from build123d import *

# Parameters (mm, degrees)
F0_W      = 340
F0_H      = 250
F1_DEPTH  = 220
F3_DEPTH  = 340
F4_R      = 110.000034
F5_DEPTH  = 228.6
F6_R      = 6.999986
F7_DEPTH  = 304.8
F8_W      = 75.12304
F8_H      = 29.99994
F9_DEPTH  = 2
F10_W     = 75
F10_H     = 30
F11_DEPTH = 2


with BuildPart() as f1:
    # F0 (on Front) → F1 (new body)
    with BuildSketch(Plane.XZ):
        Rectangle(F0_W, F0_H)
    extrude(amount=F1_DEPTH)

    # F2 (on face) → F3 (cut)
    with BuildSketch(Plane.YZ.offset(170)):
        with BuildLine():
            ThreePointArc((-40.00008, 89.98988), (-45.860908, 104.139172), (-60.0102, 110))
            Line((-60.0102, 110), (-159.98996, 110))
            ThreePointArc((-159.98996, 110), (-174.139252, 104.139172), (-180.00008, 89.98988))
            Line((-180.00008, 89.98988), (-180.00008, -89.98988))
            ThreePointArc((-180.00008, -89.98988), (-174.139252, -104.139172), (-159.98996, -110))
            Line((-159.98996, -110), (-60.0102, -110))
            ThreePointArc((-60.0102, -110), (-45.860908, -104.139172), (-40.00008, -89.98988))
            Line((-40.00008, -89.98988), (-40.00008, 89.98988))
        make_face()
    extrude(amount=-F3_DEPTH, mode=Mode.SUBTRACT)

    # F4 (on face) → F5 (cut)
    with BuildSketch(Plane.XZ.offset(220)):
        Circle(F4_R)
    extrude(amount=-F5_DEPTH, mode=Mode.SUBTRACT)

    # F6 (on face) → F7 (cut)
    with BuildSketch(Plane.XY.offset(125)):
        with Locations((0, -110.000034)):
            Circle(F6_R)
    extrude(amount=-F7_DEPTH, mode=Mode.SUBTRACT)

    # F8 (on face) → F9 (join)
    with BuildSketch(Plane(origin=(0, 0, -125), x_dir=(1, 0, 0), z_dir=(0, 0, -1))):
        with Locations((-132.43848, 205.00003)):
            Rectangle(F8_W, F8_H)
        with Locations((-132.43848, 14.99997)):
            Rectangle(F8_W, F8_H)
    extrude(amount=F9_DEPTH)

    # F10 (on face) → F11 (join)
    with BuildSketch(Plane(origin=(0, 0, -125), x_dir=(1, 0, 0), z_dir=(0, 0, -1))):
        with Locations((132.5, 110)):
            Rectangle(F10_W, F10_H)
    extrude(amount=F11_DEPTH)


solid = f1.part
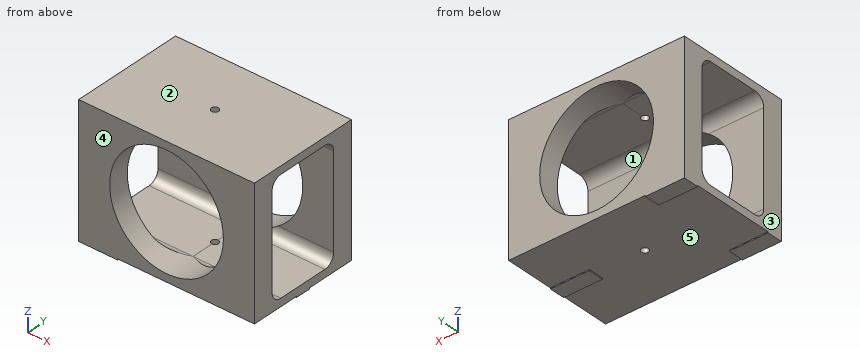
CAD build for the part. Positions are in the model's coordinates, mm. Face numbers are marked on the shaded views. A direction names the side the tool comes from. Coordinates: 2 decimals unless noted, no trailing zeros. Loops run counter-clockwise (first coordinate to the right, second up) from the corner with the lowest first, then second, coordinate; pieces in that order, holes last. Notation, with made-up numbers: (50.5, 65.25) - (57.5, 65.25) arc R4 cw to (57.5, 71.25) - close; hole circle Ø8 at (40, 22). An arc over 180 degrees is marked (long way). Write item = value, one per line. Start each with the question number.
Q1. Cut at C-C, the plane x = -11. List the corners of the cut face in (y, z), then the cut area to 3 significant figures.
Q2. Flat gauge pins, fed straight in: pin 1 Ø11 at (x, y) = (0, -110) entering from -Z; pin 2 Ø0.6 at (x, z) = (134, -126) entering from -Y; pin 3 Ø0.6 at (y, z) = (-202, -126.5) entering from +X; pin 4 Ø0.6 at (x, z) = (148.5, -126) entering from +Y. Where does each tip first touch, or does it go through?
Q3. Which spindle directions (+Z, -Z, +X, -X, +Y, -Y) get a long thin tool onto all of the face, cutting with end or side? Do the marked faces 1 and 2. Say none if no direction does.
Q4. Cut at B-B, the plane y = -143. List the corners of the cut face in (x, z), then the cut area to 3 significant figures.
Q5. Drill centre lines: L1, parallel to Y at x = 129.5, z = -87; L2, parallel to Z at x = 0, y = -178.5; L3, parallel to Y at x = 0, z = 120. Where is each one in solid material? Low to high.
Q6. Pull direction Y, two halves, no side cores. Call the marked faces 3, 4 and 5: pulls with the +Y half, pulls with the -Y half, needs draft (parallel to the pull), parting line crosses it, or undercut.
Q7. Cut at D-D, the plane z = 97.5. List the corners of the cut face in (x, y), then the cut area to 3 significant figures.
Q8. Cut at A-A, the plane z = 0. List the corners of the cut face in (x, y).
Computed:
q1.outline = (-220, -125) - (0, -125) - (0, -109.45) - (-55.35, -109.45) arc R20.01 cw to (-60.01, -110) - (-159.99, -110) arc R20.01 cw to (-164.65, -109.45) - (-220, -109.45) - close; (-220, 109.45) - (-164.65, 109.45) arc R20.01 cw to (-159.99, 110) - (-60.01, 110) arc R20.01 cw to (-55.35, 109.45) - (0, 109.45) - (0, 125) - (-220, 125) - close
q1.area = 6,730 mm²
q2.pin_1 = through
q2.pin_2 = -125
q2.pin_3 = -94.88
q2.pin_4 = -95
q3.face_1 = +X, -X
q3.face_2 = +Z, +X, -X, +Y, -Y
q4.outline = (-170, -125) - (170, -125) - (170, -110) - (0.09, -110) arc R110 cw to (-0.09, -110) - (-170, -110) - close; (-170, 110) - (-0.09, 110) arc R110 cw to (0.09, 110) - (170, 110) - (170, 125) - (-170, 125) - close
q4.area = 10,200 mm²
q5.L1 = -220 to -180, -40 to 0
q5.L2 = -125 to -110, 110 to 125
q5.L3 = -220 to -117, -103 to 0
q6.face_3 = needs draft
q6.face_4 = pulls with the -Y half
q6.face_5 = undercut
q7.outline = (-170, -220) - (-50.93, -220) - (-50.93, -178.54) - (-170, -178.54) - close; (-170, -41.46) - (-50.93, -41.46) - (-50.93, 0) - (-170, 0) - close; (50.93, -220) - (170, -220) - (170, -178.54) - (50.93, -178.54) - close; (50.93, -41.46) - (170, -41.46) - (170, 0) - (50.93, 0) - close
q7.area = 19,700 mm²
q8.outline = (-170, -220) - (-110, -220) - (-110, -180) - (-170, -180) - close; (-170, -40) - (-110, -40) - (-110, 0) - (-170, 0) - close; (110, -220) - (170, -220) - (170, -180) - (110, -180) - close; (110, -40) - (170, -40) - (170, 0) - (110, 0) - close
